CAD build for the part. Positions are in the model's coordinates, mm. A direction names the side the tool comes from. Round coordinates to 2 decimals unless told otherwise and drop trailing zeros. Order: outer loops, then holes, each group sorted by start corner. A loop starts at its lowest first (then second) coordinate and runs counter-clockwise, first axis right, second up. Notation, with made-up numbers: M 9.5,28 L 27.5,28 A14 cw 27.5,37 Z; hole C -20,-1 d10. An arc over 180 degrees is marked long. Answer as a JSON object with one key per item and string values.
```python
from build123d import *

# Parameters (mm, degrees)
BOSS_EXTRUDE1_DEPTH              = 7
F_1_8_0_125_DIAMETER_HOLE1_D     = 3.175
F_1_8_0_125_DIAMETER_HOLE1_DEPTH = 4.064
HOLE1_D                          = 15.5
F_1_4_0_25_DIAMETER_HOLE1_D      = 6.35


with BuildPart() as part:
    # Sketch1 → Boss-Extrude1 (new body)
    with BuildSketch(Plane(origin=(0, 7, 0), x_dir=(1, 0, 0), z_dir=(0, 1, 0))):
        with BuildLine():
            Line((-125.801197545, -29.648007087), (-125.801197545, 45.351992913))
            ThreePointArc((-125.801197545, 45.351992913), (-140.801197545, 60.351992913), (-155.801197545, 45.351992913))
            Line((-155.801197545, 45.351992913), (-155.801197545, -29.648007087))
            Line((-155.801197545, -29.648007087), (-125.801197545, -29.648007087))
        make_face()
    extrude(amount=-BOSS_EXTRUDE1_DEPTH)

    # 1/8 (0.125) Diameter Hole1
    with Locations(Plane(origin=(-125.801197545, 0, 0), x_dir=(0, 0, -1), z_dir=(1, 0, 0))):
        with Locations((-19.648007087, 3.5), (-9.648007087, 3.5)):
            Hole(F_1_8_0_125_DIAMETER_HOLE1_D / 2, depth=F_1_8_0_125_DIAMETER_HOLE1_DEPTH)

    # Hole1 (through all)
    with Locations(Plane(origin=(0, 0, 0), x_dir=(-1, 0, 0), z_dir=(0, -1, 0))):
        with Locations((140.801197545, -4.648007087)):
            Hole(HOLE1_D / 2)

    # 1/4 (0.25) Diameter Hole1 (through all)
    with Locations(Plane(origin=(0, 0, 0), x_dir=(-1, 0, 0), z_dir=(0, -1, 0))):
        with Locations((140.801197545, 45.351992913)):
            Hole(F_1_4_0_25_DIAMETER_HOLE1_D / 2)


solid = part.part
```
Item 1: Saw through at A-A on x = -135. List the corners of the cut face in (y, z), and give its area (3 significant figures).
Worked answers:
{"outline": "M 0,-59.18 L 7,-59.18 L 7,-0.49 L 0,-0.49 Z; M 0,9.79 L 7,9.79 L 7,29.65 L 0,29.65 Z", "area": "550 mm2"}
Item 2: Drop a flat-ended pin along its axis: pin 1 Ø1.5 at (y, z) = (3, -49.5) entering from +X. Give the stop position or say it passes through.
Worked answers:
{"pin 1": "stops at x = -126.19"}
Item 3: Wall check: line 1 along Z through (x, y) = (-137.5, 6.5); line 2 along Z through (x, y) = (-134.5, 2); line 3 along X through (y, z) = (0.5, -43). Give the ranges that are in metal, low to high. Write a range as [from, to].
Worked answers:
{"line 1": "z = [-59.98, -2.36], [11.66, 29.65]", "line 2": "z = [-58.96, 0.14], [9.16, 29.65]", "line 3": "x = [-155.8, -142.93], [-138.67, -125.8]"}
Item 4: Two-plate mould, pull along X, no slides. Class faces 1 (the cylindrical face through (-143.14, 3.55, -47.5)), 2 (the cylindrical face through (-127.862, 3.57, 8.062)), 3 (the cylindrical face through (-133.642, 3.549, 7.616)), 4 (the flat face through (-155.801, 4, -8)): released by +X, released by -X, zero draft, split by the parting line, or undercut.
Worked answers:
{"face 1": "undercut", "face 2": "zero draft", "face 3": "undercut", "face 4": "released by -X"}
Item 5: 3-axis set-ups, long thin cutter, end or side, ignore diameter. For faces 5 (the flat face through (-129.865, 4, 10)), 6 (the flat face through (-125.801, 4, -7)): which of +Z, -Z, +X, -X, +Y, -Y reach the whole face in a straight line?
Worked answers:
{"face 5": "+X", "face 6": "+Z, -Z, +X, +Y, -Y"}
Item 6: Saw through at B-B on z = -43.5. List the corners of the cut face in (x, y).
Worked answers:
{"outline": "M -155.8,0 L -143.38,0 L -143.38,7 L -155.8,7 Z; M -138.22,0 L -125.8,0 L -125.8,7 L -138.22,7 Z"}
Item 7: Saw through at C-C on y = 3.5. State how many separate pieces and enclosed holes the cut face has, and give its area (3 significant figures).
Worked answers:
{"separate pieces": "1", "enclosed holes": "2", "area": "2,360 mm2"}
